The drawing under review shows one solid part. Ordinate dimensions are in mm from its lowest x, y, z. A direction names the side the tool comes from. Give positions to 0.01 mm unless a question says otherwise; leave off trailing zeros. Write each loop counter-clockwise with the first axis right and the second up, starting at its lowest first coordinate (ties: lowest second). Pieces come first, ordered by that corner, then holes. Notation, with made-up numbers: M 78,68.25 L 96,68.25 A16 ccw 96,82.25 Z; hole C -25.5,56.25 d11. An arc over 180 degrees is marked long. One line per item, written item: value. Start each with the question number.
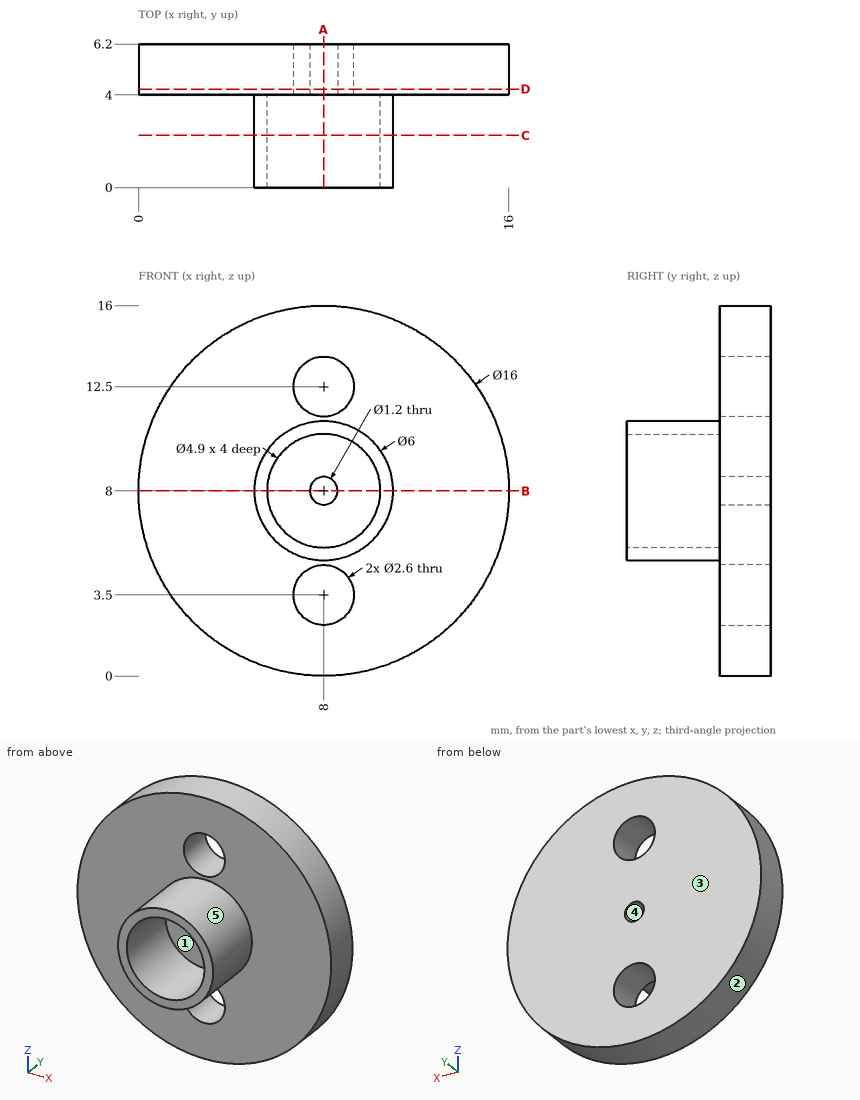
Q1. The part is to be moulded in two halves that separate along Z. For the marked faces 1, 2 and 3, say which applies: pulls with the +Z half, pulls with the -Z half, needs draft (parallel to the pull), parting line crosses it, or undercut.
Q2. Take a section at B-B, the plane z = 8. Give the boundary of the cut face in (x, y).
Q3. Take a section at D-D, the plane y = 4.25. Give the boundary of the cut face in (x, z), then the cut area to 3 significant figures.
Q4. Take a section at C-C, the plane y = 2.25. Give the boundary of the cut face in (x, z), then the cut area to 3 significant figures.
Q5. For P1, Ø3, axis at x = 6, y = 5.5, coming from the -Z side; P2, Ø1, axis at x = 8, z = 8, coming from the -Y side; P3, Ø1.5, axis at y = 2.5, z = 9, coming from the -X side, all flat-tipped, find the tip position at first contact; note any pin that passes through.
Q6. Machinability: for the marked faces 4 and 5, which of the approach directions +Z, -Z, +X, -X, +Y, -Y give a long, thin tool a straight path to every point of the face, cutting with its end or side? Answer none if there is none.
Q7. Take a section at A-A, the plane x = 8. Give the boundary of the cut face in (y, z), then the cut area to 3 significant figures.
Q8. Wall thickness on line 1 (X direction, y = 4.8, z = 8); line 2 (X direction, y = 2.1, z = 8); line 3 (Z direction, x = 7.5, y = 5.75): over which ranges is each line inside the solid? List them lowest first. Write a range as from..to.
Results list:
1. face 1: undercut
1. face 2: parting line crosses it
1. face 3: needs draft
2. outline: M 0,4 L 5,4 L 5,0 L 5.55,0 L 5.55,4 L 7.4,4 L 7.4,6.2 L 0,6.2 Z; M 8.6,4 L 10.45,4 L 10.45,0 L 11,0 L 11,4 L 16,4 L 16,6.2 L 8.6,6.2 Z
3. outline: C 8,8 d16; hole C 8,3.5 d2.6; hole C 8,12.5 d2.6; hole C 8,8 d1.2
3. area: 189 mm^2
4. outline: C 8,8 d6; hole C 8,8 d4.9
4. area: 9.42 mm^2
5. P1: stops at z = 0.02
5. P2: passes through
5. P3: stops at x = 5.01
6. face 4: +Y, -Y
6. face 5: -Y
7. outline: M 0,5 L 4,5 L 4,4.8 L 6.2,4.8 L 6.2,7.4 L 4,7.4 L 4,5.55 L 0,5.55 Z; M 0,10.45 L 4,10.45 L 4,8.6 L 6.2,8.6 L 6.2,11.2 L 4,11.2 L 4,11 L 0,11 Z; M 4,0 L 6.2,0 L 6.2,2.2 L 4,2.2 Z; M 4,13.8 L 6.2,13.8 L 6.2,16 L 4,16 Z
7. area: 25.5 mm^2
8. line 1: x = 0..7.4, 8.6..16
8. line 2: x = 5..5.55, 10.45..11
8. line 3: z = 0.02..2.3, 4.7..7.67, 8.33..11.3, 13.7..15.98
